```python
from build123d import *

# Parameters (mm, degrees)
BOSS_EXTRUDE1_DEPTH = 15
SKETCH2_R           = 9
BOSS_EXTRUDE2_DEPTH = 25
SKETCH3_W           = 130
SKETCH3_H           = 25.4
BOSS_EXTRUDE4_DEPTH = 125
CUT_EXTRUDE5_START  = -25.4
CUT_EXTRUDE5_DEPTH  = 25.4
CUT_EXTRUDE6_START  = -15.4
CUT_EXTRUDE6_DEPTH  = 15.4
SKETCH10_R          = 60
CUT_EXTRUDE9_DEPTH  = 5
SKETCH11_R          = 42.5
CUT_EXTRUDE10_DEPTH = 5
SKETCH12_R          = 2
CUT_EXTRUDE11_DEPTH = 10
SKETCH13_R          = 2
CUT_EXTRUDE12_DEPTH = 10
SKETCH14_R          = 2
CUT_EXTRUDE13_DEPTH = 10
SKETCH15_R          = 2
CUT_EXTRUDE14_DEPTH = 10


# Read off the part's stored shape, not the designer's step: Cut-Extrude5
with BuildPart() as part:
    # Sketch1 → Boss-Extrude1 (new body)
    with BuildSketch(Plane(origin=(0, 0, 0), x_dir=(1, 0, 0), z_dir=(0, 1, 0))):
        with BuildLine():
            Line((-42.755305466, 17.232797428), (94.544694534, 17.232797428))
            Line((94.544694534, 17.232797428), (94.544694534, -8.167202572))
            Line((94.544694534, -8.167202572), (-42.755305466, -8.167202572))
            ThreePointArc((-42.755305466, -8.167202572), (-55.455305466, 4.532797428), (-42.755305466, 17.232797428))
        make_face()
    extrude(amount=BOSS_EXTRUDE1_DEPTH)

    # Sketch2 → Boss-Extrude2 (add)
    with BuildSketch(Plane.XZ):
        with Locations(Location((-42.755305466, -4.532797428, 0), (0, 0, 90))):
            Circle(SKETCH2_R)
    extrude(amount=BOSS_EXTRUDE2_DEPTH)

    # Sketch3 → Boss-Extrude4 (add)
    with BuildSketch(Plane(origin=(0, 15, 0), x_dir=(1, 0, 0), z_dir=(0, 1, 0))):
        with Locations((29.544694534, 4.532797428)):
            Rectangle(SKETCH3_W, SKETCH3_H)
    extrude(amount=BOSS_EXTRUDE4_DEPTH)

    # Cut-Extrude5 outline → Cut-Extrude5 (cut)
    with BuildSketch(Plane(origin=(0, 0, -17.232797428), x_dir=(-1, 0, 0), z_dir=(0, 0, -1)).offset(CUT_EXTRUDE5_START)):
        with BuildLine():
            ThreePointArc((-94.544694534, 75), (-75.506635311, 120.961940777), (-29.544694534, 140))
            Line((-29.544694534, 140), (-94.544694534, 140))
            Line((-94.544694534, 140), (-94.544694534, 75))
        make_face()
        with BuildLine():
            ThreePointArc((-29.544694534, 140), (16.417246243, 120.961940777), (35.455305466, 75))
            Line((35.455305466, 75), (35.455305466, 140))
            Line((35.455305466, 140), (-29.544694534, 140))
        make_face()
    extrude(amount=CUT_EXTRUDE5_DEPTH, mode=Mode.SUBTRACT)

    # Sketch9 → Cut-Extrude6 (cut)
    with BuildSketch(Plane(origin=(0, 0, -17.232797428), x_dir=(-1, 0, 0), z_dir=(0, 0, -1)).offset(CUT_EXTRUDE6_START)):
        with BuildLine():
            Line((35.455305466, 15), (-94.544694534, 15))
            Line((-94.544694534, 15), (-94.544694534, 75))
            ThreePointArc((-94.544694534, 75), (-29.544694534, 140), (35.455305466, 75))
            Line((35.455305466, 75), (35.455305466, 15))
        make_face()
    extrude(amount=CUT_EXTRUDE6_DEPTH, mode=Mode.SUBTRACT)

    # Sketch10 → Cut-Extrude9 (cut)
    with BuildSketch(Plane(origin=(0, 0, -1.832797428), x_dir=(-1, 0, 0), z_dir=(0, 0, -1))):
        with Locations((-29.544694534, 75)):
            Circle(SKETCH10_R)
    extrude(amount=-CUT_EXTRUDE9_DEPTH, mode=Mode.SUBTRACT)

    # Sketch11 → Cut-Extrude10 (cut)
    with BuildSketch(Plane(origin=(0, 0, 3.167202572), x_dir=(-1, 0, 0), z_dir=(0, 0, -1))):
        with Locations((-29.544694534, 75)):
            Circle(SKETCH11_R)
    extrude(amount=-CUT_EXTRUDE10_DEPTH, mode=Mode.SUBTRACT)

    # Sketch12 → Cut-Extrude11 (cut)
    with BuildSketch(Plane(origin=(0, 0, 3.167202572), x_dir=(-1, 0, 0), z_dir=(0, 0, -1))):
        with Locations((-29.544694534, 123)):
            Circle(SKETCH12_R)
        with Locations((4.26307508, 108.619175914)):
            Circle(SKETCH12_R)
        with Locations((18, 74.544694534)):
            Circle(SKETCH12_R)
        with Locations((3.619175914, 40.73692492)):
            Circle(SKETCH12_R)
        with Locations((-30.455305466, 27)):
            Circle(SKETCH12_R)
        with Locations((-64.26307508, 41.380824086)):
            Circle(SKETCH12_R)
        with Locations((-78, 75.455305466)):
            Circle(SKETCH12_R)
        with Locations((-63.619175914, 109.26307508)):
            Circle(SKETCH12_R)
    extrude(amount=-CUT_EXTRUDE11_DEPTH, mode=Mode.SUBTRACT)

    # Sketch13 → Cut-Extrude12 (cut)
    with BuildSketch(Plane(origin=(0, 0, -1.832797428), x_dir=(-1, 0, 0), z_dir=(0, 0, -1))):
        with Locations((-89.544694534, 25)):
            Circle(SKETCH13_R)
        with Locations((30.455305466, 25)):
            Circle(SKETCH13_R)
    extrude(amount=-CUT_EXTRUDE12_DEPTH, mode=Mode.SUBTRACT)

    # Sketch14 → Cut-Extrude13 (cut)
    with BuildSketch(Plane(origin=(0, 0, -1.832797428), x_dir=(-1, 0, 0), z_dir=(0, 0, -1))):
        with Locations((-91.944694534, 74.269730636)):
            Circle(SKETCH14_R)
        with Locations((32.855305466, 74.269730636)):
            Circle(SKETCH14_R)
    extrude(amount=-CUT_EXTRUDE13_DEPTH, mode=Mode.SUBTRACT)

    # Sketch15 → Cut-Extrude14 (cut)
    with BuildSketch(Plane(origin=(0, 0, -1.832797428), x_dir=(-1, 0, 0), z_dir=(0, 0, -1))):
        with Locations((-29.607268832, 137.499968676)):
            Circle(SKETCH15_R)
    extrude(amount=-CUT_EXTRUDE14_DEPTH, mode=Mode.SUBTRACT)


solid = part.part
```
Could you check a few things on this model? Use its own coordinates, in mm. A direction names the side the tool comes from. Coordinates: 2 decimals unless noted, no trailing zeros. Loops run counter-clockwise (first coordinate to the right, second up) from the corner with the lowest first, then second, coordinate; pieces in that order, holes last. Notation, with made-up numbers: M 66.5,64.5 L 88.5,64.5 A18 cw 88.5,73.5 Z; hole C 10,17.5 d7. An arc over 180 degrees is marked long. Put each result on its own line as item: value. Start each with the question number.
(1) Will these pins go through, and if not, where does the flat tip stop? P1, Ø12, axis at y = 105, z = -0.5, coming from the +X side; P2, Ø1, axis at x = 21, z = -12.5, coming from the +Y side; P3, Ø3.5, axis at x = 91.94, y = 74.27, coming from the +Z side; P4, Ø1, axis at x = -14, z = 5, coming from the -Y side.
(2) Thinking about a two-plate mould opening in X: for faces 5 (the face through (21, 15, -8)), 6 (the face through (-34.77, -12.32, -0.38)), 7 (the face through (-55.452, 7.395, -4.254)), 8 (the face through (91.13, 23.78, 3.1)), which applies, pulls with the +X half, pulls with the -X half, needs draft (parallel to the pull), parting line crosses it, or undercut?
(3) Suppose I cut it at C-C on z = 0. Please give me the cut outline in (x, y).
(4) Suppose I cut it at D-D on z = -11.5. Please give me the cut outline in (x, y).
(5) Suppose I cut it at A-A on y = 90.5. Please give me the cut outline in (x, z), then the cut area to 3 significant figures.
(6) I need wall thicknesses on line 1 (Y direction, x = -43.5, z = -11.5); line 2 (Y direction, x = -6, z = -9.75); line 3 (Z direction, x = 86, y = 103). Which ranges of each line are inside material? Lowest first, please. Write a range as from..to.
(7) For faces 1 (the face through (10, 18, -1.833)), 2 (the face through (70.4, 62.5, 3.167)), 3 (the face through (-35.455, 45, 3)), 4 (the face through (-3.83, 106.667, 5.632)), which set-ups out of +Z, -Z, +X, -X, +Y, -Y let a thin tool reach every point of the face, with its end or its side?
(8) Suppose I cut it at B-B on x = 36.5. Please give me the cut outline in (y, z).
Solutions:
1. P1: stops at x = 89.95
1. P2: stops at y = 15
1. P3: passes through
1. P4: stops at y = 0
2. face 5: needs draft
2. face 6: parting line crosses it
2. face 7: pulls with the -X half
2. face 8: undercut
3. outline: M -54.62,0 L -50.53,0 L -50.53,-25 L -34.98,-25 L -34.98,0 L 94.54,0 L 94.54,75 A65 ccw -35.46,75 L -35.46,15 L -54.62,15 Z; hole C -32.86,74.27 d4; hole C -30.46,25 d4; hole C 29.54,75 d120; hole C 29.61,137.5 d4; hole C 89.54,25 d4; hole C 91.94,74.27 d4
4. outline: M -53.37,0 L -48.45,0 L -48.45,-25 L -37.06,-25 L -37.06,0 L 94.54,0 L 94.54,15 L -53.37,15 Z
5. outline: M -33.58,-1.83 L -28.42,-1.83 L -28.42,3.17 L -10.03,3.17 L -10.03,8.17 L -33.58,8.17 Z; M 69.12,3.17 L 87.51,3.17 L 87.51,-1.83 L 92.67,-1.83 L 92.67,8.17 L 69.12,8.17 Z
5. area: 287 mm2
6. line 1: y = -25..15
6. line 2: y = 0..15
6. line 3: z = -1.83..8.17
7. face 1: -Z, +X, -X, +Y
7. face 2: -Z
7. face 3: +Z, -Z, -X, +Y
7. face 4: +Z, -Z
8. outline: M 0,-17.23 L 15,-17.23 L 15,-1.83 L 15.4,-1.83 L 15.4,3.17 L 33.07,3.17 L 33.07,8.17 L 0,8.17 Z; M 116.93,3.17 L 134.6,3.17 L 134.6,-1.83 L 139.63,-1.83 L 139.63,8.17 L 116.93,8.17 Z
